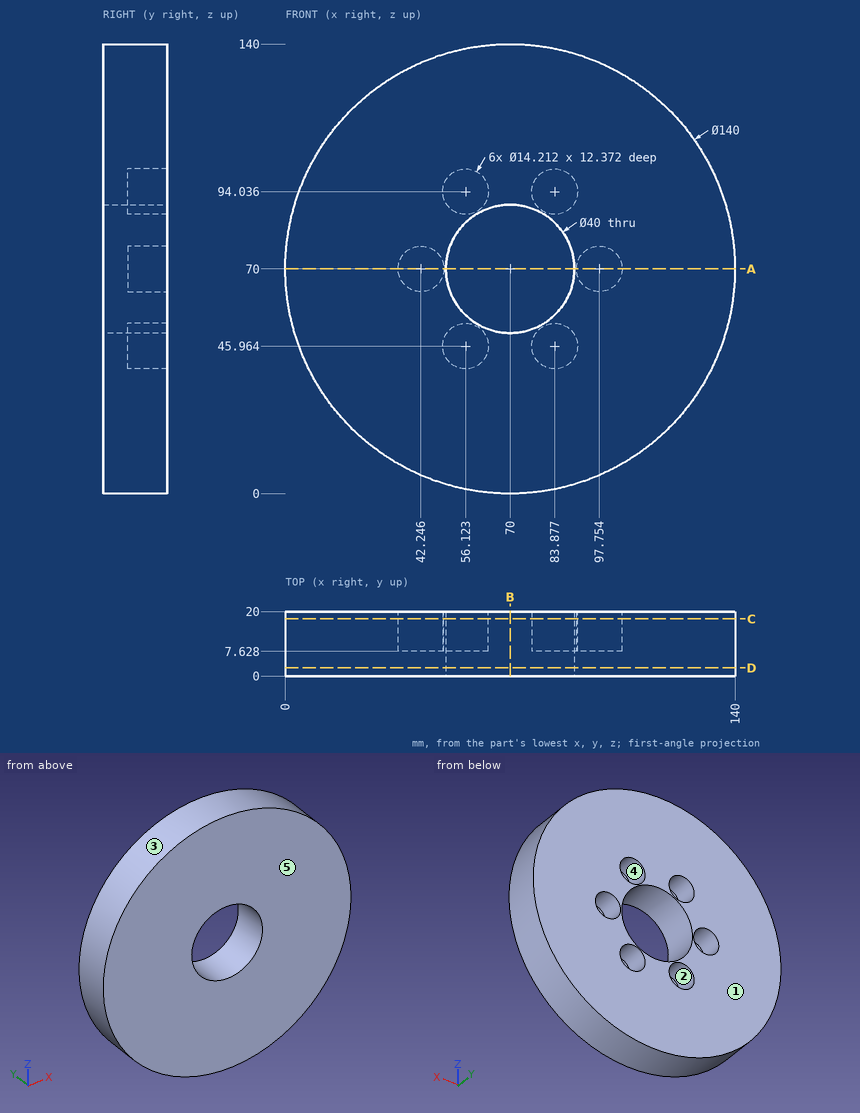
For this review, use the dimensioned drawing (mm, ordinates from the lowest corner) and the shaded views. A direction names the side the tool comes from. Round coordinates to 2 decimals unless told otherwise and drop trailing zeros. Write each loop counter-clockwise with the first axis right and the second up, starting at its lowest first coordinate (ties: lowest second). Pieces come first, ordered by that corner, then holes. Notation, with made-up numbers: M 52,2.25 L 76,2.25 A29 cw 76,41.25 Z; hole C -9,-27.75 d2. An arc over 180 degrees is marked long. Use CSV: the item, a comma, the result in double quotes. Start each with the question number.
(1) We need section B-B, the plane x = 70. State the section outline as (y, z) points.
(2) For line 1 along X through (y, z) = (17.25, 70); line 2 along Y through (x, z) = (88, 90); line 3 along X through (y, z) = (11, 40) (1 decimal), list the stretches that pass through material, from the lowest coordinate up.
(3) Tool access review of the marked faces 4 and 5: name each direction out of +Z, -Z, +X, -X, +Y, -Y from which nothing blocks a thin tool from reaching the whole face with its end or side.
(4) Clearance check with flat-ended pins moving along their axes: P1, Ø24, axis at x = 70, z = 70, coming from the +Y side; P2, Ø11.5, axis at x = 85, z = 46.5, coming from the +Y side; P3, Ø5, axis at y = 9.5, z = 123, coming from the -X side (1 decimal); P4, Ø3, axis at y = 18, z = 42.5, coming from the -X side. State where each tip first meets the part, or that it passes through.
(5) We need section D-D, the plane y = 2.5. State the section outline as (x, z) points, then the cut area to 3 significant figures.
(6) The part is to be moulded in two halves that separate along X. For the marked faces 1, 2 and 3, say which applies: +X half, -X half, draft (parallel to the pull), parting line (faces both ways), or undercut.
(7) We need section C-C, the plane y = 17.75. State the section outline as (x, z) points (1 decimal).
(8) We need section A-A, the plane z = 70. State the section outline as (x, y) points, then the cut area to 3 significant figures.
Findings:
1,outline,"M 0,0 L 20,0 L 20,50 L 0,50 Z; M 0,90 L 20,90 L 20,140 L 0,140 Z"
2,line 1,"0 to 35.14, 49.35 to 50, 90 to 90.65, 104.86 to 140"
2,line 2,"0 to 7.63"
2,line 3,"6.8 to 52.3, 60 to 80, 87.7 to 133.2"
3,face 4,"+Y"
3,face 5,"+Z, -Z, +X, -X, -Y"
4,P1,"through"
4,P2,"y = 7.63"
4,P3,"x = 21.5"
4,P4,"x = 5.01"
5,outline,"C 70,70 d140; hole C 70,70 d40"
5,area,"14,100 mm^2"
6,face 1,"draft"
6,face 2,"undercut"
6,face 3,"parting line"
7,outline,"C 70,70 d140; hole C 42.2,70 d14.2; hole C 56.1,46 d14.2; hole C 56.1,94 d14.2; hole C 70,70 d40; hole C 83.9,46 d14.2; hole C 83.9,94 d14.2; hole C 97.8,70 d14.2"
8,outline,"M 0,0 L 50,0 L 50,20 L 49.35,20 L 49.35,7.63 L 35.14,7.63 L 35.14,20 L 0,20 Z; M 90,0 L 140,0 L 140,20 L 104.86,20 L 104.86,7.63 L 90.65,7.63 L 90.65,20 L 90,20 Z"
8,area,"1,650 mm^2"
